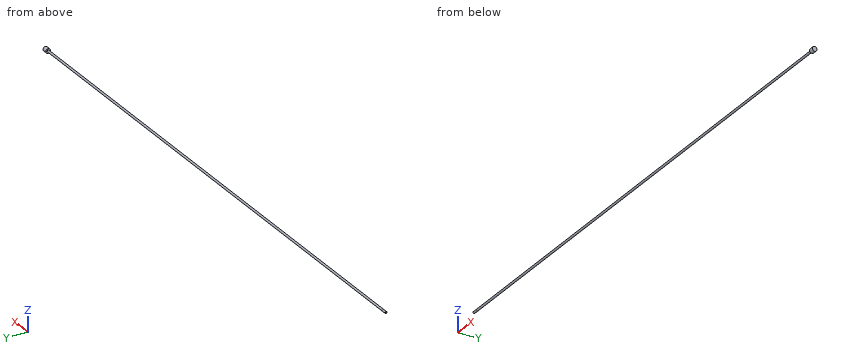
from build123d import *

# Parameters (mm, degrees)
SKETCH3_W = 0.254
SKETCH3_H = 0.508


with BuildPart() as part:
    # Sketch1 → Revolve1 (revolve)
    with BuildSketch(Plane.XY):
        Polygon((0, 0), (0, 2.3749), (1300.1752, 2.3749), (1300.1752, 5.61975), (1311.1988, 5.61975), (1311.1988, 0), align=None)
    revolve(axis=Axis((1311.1988, 0, 0), (-1, 0, 0)))

    # Sketch2 → Revolve2 (revolve)
    with BuildSketch(Plane.XY):
        Polygon((-12.7, 0), (-12.7, 1.94056), (-12.22756, 2.413), (0, 2.413), (0, 0), align=None)
    revolve(axis=Axis((0, 0, 0), (-1, 0, 0)))

    # Sketch3 → Cut-Revolve1 (revolve, cut)
    with BuildSketch(Plane.XY):
        with Locations((-0.127, 2.413)):
            Rectangle(SKETCH3_W, SKETCH3_H)
    revolve(axis=Axis((0, 0, 0), (-1, 0, 0)), mode=Mode.SUBTRACT)


solid = part.part
Build history of the part. All positions in model axes, mm. Give positions to 0.01 mm unless a question says otherwise; leave off trailing zeros. Order: outer loops, then holes, each group sorted by start corner. A loop starts at its lowest first (then second) coordinate and runs counter-clockwise, first axis right, second up. Notation, with made-up numbers: M 27,-19.75 L 37,-19.75 A22 cw 37,-3.75 Z; hole C 85,80.5 d1. An arc over 180 degrees is marked long. Use one line per item in the form item = value.
Q1. Pin check, flat tips, straight feed: P1, Ø4, axis at y = -2, z = -4, coming from the -X side; P2, Ø2, axis at x = 837, y = 1, coming from the -Z side; P3, Ø6, axis at x = 413, z = -2, coming from the +Y side. Stop position of each tip, or through.
Conclusion:
P1 = 1300.18
P2 = -2.37
P3 = 2.37
Q2. Slice it at C-C, the plane x = 992. Write the cut outline in (y, z), and give its area (3 significant figures).
Conclusion:
outline = C 0,0 d4.75
area = 17.7 mm2
Q3. Slice it at A-A, the plane y = 0. Write the cut outline in (x, z), and give its area (3 significant figures).
Conclusion:
outline = M -12.7,-1.94 L -12.23,-2.41 L -0.25,-2.41 L -0.25,-2.16 L 0,-2.16 L 0,-2.37 L 1300.18,-2.37 L 1300.18,-5.62 L 1311.2,-5.62 L 1311.2,5.62 L 1300.18,5.62 L 1300.18,2.37 L 0,2.37 L 0,2.16 L -0.25,2.16 L -0.25,2.41 L -12.23,2.41 L -12.7,1.94 Z
area = 6,360 mm2
Q4. Wall check: probe 1 along Z at (x, y) = (532, -1); probe 2 along Z at (x, y) = (43, 0.5); probe 3 along X at (y, z) = (-0.5, -3.75). Give the ranges that are in metal, low to high.
Conclusion:
probe_1 = -2.15 to 2.15
probe_2 = -2.32 to 2.32
probe_3 = 1300.18 to 1311.2
